```python
from build123d import *

# Parameters (mm, degrees)
F1_DEPTH = 6.35
F3_DEPTH = 12.7
F5_DEPTH = 12.7
F6_R     = 6.35
F7_DEPTH = 25.4
F8_R     = 3.175
F9_DEPTH = 6.35


with BuildPart() as f1:
    # F0 (on Top) → F1 (new body)
    with BuildSketch(Plane.XY):
        with BuildLine():
            Line((50.8, 0), (0, 0))
            Line((0, 0), (0, -25.4))
            ThreePointArc((0, -25.4), (6.35, -19.05), (12.7, -25.4))
            Line((12.7, -25.4), (38.1, -25.4))
            ThreePointArc((38.1, -25.4), (44.45, -19.05), (50.8, -25.4))
            Line((50.8, -25.4), (50.8, 0))
        make_face()
        with BuildLine():
            ThreePointArc((12.7, -25.4), (6.35, -19.05), (0, -25.4))
            Line((0, -25.4), (6.35, -25.4))
            Line((6.35, -25.4), (12.7, -25.4))
        make_face()
        with BuildLine():
            Line((6.35, -25.4), (0, -25.4))
            ThreePointArc((0, -25.4), (1.8598719395, -29.8901280605), (6.35, -31.75))
            Line((6.35, -31.75), (6.35, -25.4))
        make_face()
        with BuildLine():
            Line((12.7, -25.4), (6.35, -25.4))
            Line((6.35, -25.4), (6.35, -31.75))
            ThreePointArc((6.35, -31.75), (10.8401280605, -29.8901280605), (12.7, -25.4))
        make_face()
        with BuildLine():
            Line((38.1, -25.4), (12.7, -25.4))
            ThreePointArc((12.7, -25.4), (10.8401280605, -29.8901280605), (6.35, -31.75))
            Line((6.35, -31.75), (44.45, -31.75))
            ThreePointArc((44.45, -31.75), (39.9598719395, -29.8901280605), (38.1, -25.4))
        make_face()
        with BuildLine():
            Line((44.45, -31.75), (44.45, -25.4))
            Line((44.45, -25.4), (38.1, -25.4))
            ThreePointArc((38.1, -25.4), (39.9598719395, -29.8901280605), (44.45, -31.75))
        make_face()
        with BuildLine():
            ThreePointArc((44.45, -31.75), (48.9401280605, -29.8901280605), (50.8, -25.4))
            Line((50.8, -25.4), (44.45, -25.4))
            Line((44.45, -25.4), (44.45, -31.75))
        make_face()
        with BuildLine():
            Line((44.45, -25.4), (50.8, -25.4))
            ThreePointArc((50.8, -25.4), (44.45, -19.05), (38.1, -25.4))
            Line((38.1, -25.4), (44.45, -25.4))
        make_face()
    extrude(amount=F1_DEPTH)

    # F2 (on Front) → F3 (join)
    with BuildSketch(Plane.XZ):
        with BuildLine():
            Line((12.7, 19.05), (12.7, 6.35))
            Line((12.7, 6.35), (38.1, 6.35))
            Line((38.1, 6.35), (38.1, 19.05))
            Line((38.1, 19.05), (38.1, 50.8))
            ThreePointArc((38.1, 50.8), (25.4, 38.1), (12.7, 50.8))
            Line((12.7, 50.8), (12.7, 19.05))
        make_face()
        with BuildLine():
            Line((0, 6.35), (12.7, 6.35))
            Line((12.7, 6.35), (12.7, 19.05))
            ThreePointArc((12.7, 19.05), (8.9802561211, 10.0697438789), (0, 6.35))
        make_face()
        with BuildLine():
            Line((38.1, 19.05), (38.1, 6.35))
            Line((38.1, 6.35), (50.8, 6.35))
            ThreePointArc((50.8, 6.35), (41.8197438789, 10.0697438789), (38.1, 19.05))
        make_face()
        with BuildLine():
            ThreePointArc((38.1, 50.8), (25.4, 63.5), (12.7, 50.8))
            Line((12.7, 50.8), (38.1, 50.8))
        make_face()
        with BuildLine():
            Line((38.1, 50.8), (12.7, 50.8))
            ThreePointArc((12.7, 50.8), (25.4, 38.1), (38.1, 50.8))
        make_face()
    extrude(amount=F3_DEPTH)

    # F4 (on face) → F5 (join)
    with BuildSketch(Plane.XZ.offset(12.7)):
        with BuildLine():
            ThreePointArc((12.7, 50.8), (25.4, 38.1), (38.1, 50.8))
            ThreePointArc((38.1, 50.8), (25.4, 63.5), (12.7, 50.8))
        make_face()
    extrude(amount=F5_DEPTH)

    # F6 (on face) → F7 (cut)
    with BuildSketch(Plane.XZ.offset(25.4)):
        with Locations((25.4, 50.8)):
            Circle(F6_R)
    extrude(amount=-F7_DEPTH, mode=Mode.SUBTRACT)

    # F8 (on face) → F9 (cut)
    with BuildSketch(Plane.XY.offset(6.35)):
        with Locations((9.525, -22.225)):
            Circle(F8_R)
        with Locations((41.275, -22.225)):
            Circle(F8_R)
    extrude(amount=-F9_DEPTH, mode=Mode.SUBTRACT)


solid = f1.part
```
CAD build for the part. Positions are in the model's coordinates, mm. A direction names the side the tool comes from. Round coordinates to 2 decimals unless told otherwise and drop trailing zeros. Order: outer loops, then holes, each group sorted by start corner. A loop starts at its lowest first (then second) coordinate and runs counter-clockwise, first axis right, second up. Notation, with made-up numbers: (53, 9) -> (64, 9) arc R19 ccw to (64, 45) -> close; hole circle Ø4 at (-7, 50). An arc over 180 degrees is marked (long way). Write item = value, one per line.
(1) 3-axis set-ups, long thin cutter, end or side, ignore diameter. For faces 4 (the flat face through (12.7, -6, 35)), 5 (the flat face through (38.1, -6, 35)), 6 (the flat face through (28, -25.4, 57)): which of +Z, -Z, +X, -X, +Y, -Y reach the whole face in a straight line?
Answers follow:
face_4 = +Z, -X, +Y, -Y
face_5 = +Z, +X, +Y, -Y
face_6 = +Z, +X, -X, -Y
(2) Pull direction Z, two halves, no side cores. Call faces 1 (the flat face through (25, -12.7, 24)), 2 (the cylindrical face through (41.92, -6.26, 9.97)), 3 (the flat face through (25, -31.75, 3)): +Z half, -Z half, draft (parallel to the pull), parting line (faces both ways), or undercut.
Answers follow:
face_1 = undercut
face_2 = +Z half
face_3 = draft
(3) Cut at A-A (y = -17.5). Write the cut outline in (x, z).
Answers follow:
outline = (0, 0) -> (50.8, 0) -> (50.8, 6.35) -> (0, 6.35) -> close; circle Ø25.4 at (25.4, 50.8); hole circle Ø12.7 at (25.4, 50.8)
(4) Drill centre lines: L1, parallel to Z at x = 25, y = -16; L2, parallel to Z at x = 25.4, y = -7.5; L3, parallel to X at y = -19, z = 51. Where is each one in solid material? Low to high.
Answers follow:
L1 = 0 to 6.35, 38.11 to 44.46, 57.14 to 63.49
L2 = 0 to 44.45, 57.15 to 63.5
L3 = 12.7 to 19.05, 31.75 to 38.1
(5) Cut at D-D (x = 7.5). Write the cut outline in (y, z), plus the area to 3 significant figures.
Answers follow:
outline = (-31.75, 0) -> (-24.67, 0) -> (-24.67, 6.35) -> (-31.75, 6.35) -> close; (-19.78, 0) -> (0, 0) -> (0, 8.8) -> (-12.7, 8.8) -> (-12.7, 6.35) -> (-19.78, 6.35) -> close
area = 202 mm²
(6) Flat gauge pins, fed straight in: P1, Ø13.5, axis at x = 17, z = 33.5, coming from the -Y side; P2, Ø12, axis at x = 38.5, y = -17.5, coming from the +Z side; P3, Ø14, axis at y = -6, z = 28.5, coming from the -X side; P4, Ø5.5, axis at x = 41.275, y = -22.225, coming from the +Z side. Where does each tip first touch, or does it go through?
Answers follow:
P1 = -25.4
P2 = 61.33
P3 = 12.7
P4 = through
(7) Cut at B-B (x = 25.4). Write the cut outline in (y, z), plus the area to 3 significant figures.
Answers follow:
outline = (-31.75, 0) -> (0, 0) -> (0, 44.45) -> (-25.4, 44.45) -> (-25.4, 38.1) -> (-12.7, 38.1) -> (-12.7, 6.35) -> (-31.75, 6.35) -> close; (-25.4, 57.15) -> (0, 57.15) -> (0, 63.5) -> (-25.4, 63.5) -> close
area = 927 mm²
(8) Cut at C-C (y = -4.5). Write the cut outline in (x, z), plus the area to 3 significant figures.
Answers follow:
outline = (0, 0) -> (50.8, 0) -> (50.8, 6.35) arc R12.7 cw to (38.1, 19.05) -> (38.1, 50.8) arc R12.7 ccw to (12.7, 50.8) -> (12.7, 19.05) arc R12.7 cw to (0, 6.35) -> close; hole circle Ø12.7 at (25.4, 50.8)
area = 1,650 mm²
